from build123d import *

# Parameters (mm, degrees)
F0_R     = 4
F1_DEPTH = 45
F2_R     = 6
F3_DEPTH = 35
F7_R     = 0.5
F8_SIZE  = 0.5


with BuildPart() as f1:
    # F0 (on Right) → F1 (new body, symmetric)
    with BuildSketch(Plane.YZ):
        Circle(F0_R)
    extrude(amount=F1_DEPTH, both=True)

    # F2 (on Right) → F3 (join, symmetric)
    with BuildSketch(Plane.YZ):
        Circle(F2_R)
    extrude(amount=F3_DEPTH, both=True)

    # F4 (on Front) → F6 (revolve, cut)
    with BuildSketch(Plane.XZ):
        with BuildLine():
            Line((30, 6), (-30, 6))
            ThreePointArc((-30, 6), (0, 4), (30, 6))
        make_face()
    revolve(axis=Axis((12.5838983804, 0, 0), (1, 0, 0)), mode=Mode.SUBTRACT)

    # F7
    f7_edges = [f1.edges().sort_by_distance(p)[0] for p in [
        (-35, -6, 0),
        (35, -6, 0),
    ]]
    fillet(f7_edges, radius=F7_R)

    # F8
    f8_edges = [f1.edges().sort_by_distance(p)[0] for p in [
        (-45, -4, 0),
        (45, -4, 0),
    ]]
    chamfer(f8_edges, length=F8_SIZE)


solid = f1.part
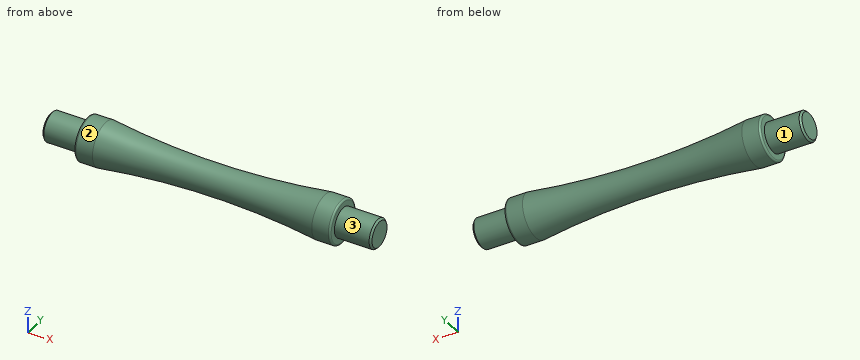
The listing builds one solid part. Answer for the finished solid, in the listing's coordinates (mm). Face numbers are marked on the shaded views. A direction names the side the tool comes from. Give positions to 0.01 mm unless a question says otherwise; leave off trailing zeros. Write each loop counter-clockwise with the first axis right and the second up, starting at its lowest first coordinate (ties: lowest second). Pieces come first, ordered by that corner, then holes. Notation, with made-up numbers: (20, 84) - (28, 84) arc R28 cw to (28, 122) - close; hole circle Ø2 at (79, 39). An arc over 180 degrees is marked (long way). Use a Markdown table: item, result.
1. Section A-A on y = 0 is taken. Write down the section's boundary in (x, z).
Values follow:
| item | result |
|---|---|
| outline | (-45, -3.5) - (-44.5, -4) - (-35, -4) - (-35, -5.5) arc R0.5 ccw to (-34.5, -6) - (-30, -6) arc R226 cw to (30, -6) - (34.5, -6) arc R0.5 ccw to (35, -5.5) - (35, -4) - (44.5, -4) - (45, -3.5) - (45, 3.5) - (44.5, 4) - (35, 4) - (35, 5.5) arc R0.5 ccw to (34.5, 6) - (30, 6) arc R226 cw to (-30, 6) - (-34.5, 6) arc R0.5 ccw to (-35, 5.5) - (-35, 4) - (-44.5, 4) - (-45, 3.5) - close |
2. A tool of negligible diameter and unlimited length cuts with its end or side. For the marked faces 1, 2 and 3, from which of +Z, -Z, +X, -X, +Y, -Y can it reach the whole face along a straight path? Write none if from no direction.
Values follow:
| item | result |
|---|---|
| face 1 | -X |
| face 2 | +X, -X |
| face 3 | +X |
3. Section C-C on x = -15 is taken. Write down the section's boundary in (y, z).
Values follow:
| item | result |
|---|---|
| outline | circle Ø9 at (0, 0) |
4. Section D-D on x = 1 is taken. Write down the section's boundary in (y, z).
Values follow:
| item | result |
|---|---|
| outline | circle Ø8 at (0, 0) |
5. Each of these flat-tipped pins is pushed along its axis until it touches: P1, Ø1, axis at x = -15.5, y = 3.5, coming from the +Z side; P2, Ø1.5, axis at x = -9.5, z = 0, coming from the -Y side; P3, Ø1.5, axis at x = -33.5, z = 4.5, coming from the +Y side. Where does it stop, or does it pass through?
Values follow:
| item | result |
|---|---|
| P1 | stops at z = 3.4 |
| P2 | stops at y = -4.23 |
| P3 | stops at y = 4.68 |
6. Find the intervals of material crossed by probe 1 along Z at (x, y) = (-11, 1.5); probe 2 along Y at (x, z) = (-32, -1.75); probe 3 along Z at (x, y) = (19, -0.5), in increasing order. Write a range as from..to.
Values follow:
| item | result |
|---|---|
| probe 1 | z = -4..4 |
| probe 2 | y = -5.74..5.74 |
| probe 3 | z = -4.77..4.77 |
